The listing builds one solid part. Answer for the finished solid, in the listing's coordinates (mm). A direction names the side the tool comes from. Round coordinates to 2 decimals unless told otherwise and drop trailing zeros. Loops run counter-clockwise (first coordinate to the right, second up) from the corner with the lowest first, then second, coordinate; pieces in that order, holes last. Notation, with made-up numbers: M 2,88 L 52,88 A21 ccw 52,121 Z; hole C 24,-18.75 d6. An arc over 180 degrees is marked long. Answer as a JSON object with one key per item and string values.
```python
from build123d import *

# Parameters (mm, degrees)
SKETCH1_W           = 11
SKETCH1_H           = 11
BOSS_EXTRUDE1_DEPTH = 3


with BuildPart() as part:
    # Sketch1 → Boss-Extrude1 (new body)
    with BuildSketch(Plane.XY):
        with BuildLine():
            Line((0, 0), (88, 0))
            Line((88, 0), (88, 17))
            ThreePointArc((88, 17), (86.535533906, 20.535533906), (83, 22))
            Line((83, 22), (5, 22))
            ThreePointArc((5, 22), (1.464466094, 20.535533906), (0, 17))
            Line((0, 17), (0, 0))
        make_face()
        with Locations((10.5, 11.7)):
            Rectangle(SKETCH1_W, SKETCH1_H, mode=Mode.SUBTRACT)
        with Locations((29.5, 11.7)):
            Rectangle(SKETCH1_W, SKETCH1_H, mode=Mode.SUBTRACT)
        with Locations((48.5, 11.7)):
            Rectangle(SKETCH1_W, SKETCH1_H, mode=Mode.SUBTRACT)
        with Locations((67.5, 11.7)):
            Rectangle(SKETCH1_W, SKETCH1_H, mode=Mode.SUBTRACT)
    extrude(amount=BOSS_EXTRUDE1_DEPTH)


solid = part.part
```
Item 1: The part is cut by section C-C (z = 0.6). Give the vertices of the cut face in (x, y).
Values follow:
{"outline": "M 0,0 L 88,0 L 88,17 A5 ccw 83,22 L 5,22 A5 ccw 0,17 Z; hole M 5,6.2 L 16,6.2 L 16,17.2 L 5,17.2 Z; hole M 24,6.2 L 35,6.2 L 35,17.2 L 24,17.2 Z; hole M 43,6.2 L 54,6.2 L 54,17.2 L 43,17.2 Z; hole M 62,6.2 L 73,6.2 L 73,17.2 L 62,17.2 Z"}
Item 2: The part is cut by section B-B (x = 6). Give the vertices of the cut face in (y, z), then the cut area to 3 significant figures.
Values follow:
{"outline": "M 0,0 L 6.2,0 L 6.2,3 L 0,3 Z; M 17.2,0 L 22,0 L 22,3 L 17.2,3 Z", "area": "33.0 mm^2"}
Item 3: The part is cut by section A-A (y = 7.5). Give the vertices of the cut face in (x, z), then the cut area to 3 significant figures.
Values follow:
{"outline": "M 0,0 L 5,0 L 5,3 L 0,3 Z; M 16,0 L 24,0 L 24,3 L 16,3 Z; M 35,0 L 43,0 L 43,3 L 35,3 Z; M 54,0 L 62,0 L 62,3 L 54,3 Z; M 73,0 L 88,0 L 88,3 L 73,3 Z", "area": "132 mm^2"}
Item 4: Determine the mould class of faces 3 (the face through (0, 9, 1)), 4 (the face through (87, 20, 1)), 5 (the face through (48, 17.2, 1)) for opening direction Y: released by +Y, released by -Y, zero draft, split by the parting line, or undercut.
Values follow:
{"face 3": "zero draft", "face 4": "released by +Y", "face 5": "undercut"}
Item 5: Which of the six approach directions +Z, -Z, +X, -X, +Y, -Y give full straight-line access (tool end or side, diameter ignored) to faces 1 (the face through (43, 18, 3)), 2 (the face through (73, 12, 1))?
Values follow:
{"face 1": "+Z, +X, -X, +Y, -Y", "face 2": "+Z, -Z"}
Item 6: The part is cut by section D-D (y = 20). Give the vertices of the cut face in (x, z), then the cut area to 3 significant figures.
Values follow:
{"outline": "M 1,0 L 87,0 L 87,3 L 1,3 Z", "area": "258 mm^2"}
Item 7: Straight lines are drawn through the part: line 1 (X direction, y = 7.75, z = 2.75); line 2 (Y direction, x = 63.5, z = 0.7); line 3 (X direction, y = 17.25, z = 2.4). For each, find the intervals that lie inside material, in ascending order.
Values follow:
{"line 1": "0 to 5, 16 to 24, 35 to 43, 54 to 62, 73 to 88", "line 2": "0 to 6.2, 17.2 to 22", "line 3": "0.01 to 87.99"}
